Could you check a few things on this model? Use its own coordinates, in mm. A direction names the side the tool comes from. Round coordinates to 2 decimals unless told otherwise and drop trailing zeros. Loops run counter-clockwise (first coordinate to the right, second up) from the corner with the lowest first, then second, coordinate; pieces in that order, holes last. Notation, with made-up numbers: (-18, 56.5) - (1, 56.5) arc R21 ccw to (1, 81.5) - close; hole circle Ø7 at (84.5, 9.5). An arc over 180 degrees is marked (long way). Put each result on its own line as item: value. Start each with the question number.
from build123d import *

# Parameters (mm, degrees)
SKETCH1_R               = 75
BOSS_EXTRUDE1_DEPTH     = 50
CUT_EXTRUDE1_DEPTH      = 290.39592257
CUT_EXTRUDE1_DEPTH_BACK = 290.39592257
FILLET1_START           = -50
FILLET1_DEPTH           = 100


with BuildPart() as part:
    # Sketch1 → Boss-Extrude1 (new, symmetric)
    with BuildSketch(Plane.XY):
        with BuildLine():
            Line((-95.945006832, -117.34375), (-36.550478793, 16.25))
            ThreePointArc((-36.550478793, 16.25), (0, 40), (36.550478793, 16.25))
            Line((36.550478793, 16.25), (95.945006832, -117.34375))
            ThreePointArc((95.945006832, -117.34375), (0, -265), (-95.945006832, -117.34375))
        make_face()
        with Locations((0, -160)):
            Circle(SKETCH1_R, mode=Mode.SUBTRACT)
    extrude(amount=BOSS_EXTRUDE1_DEPTH, both=True)

    # Sketch2 → Cut-Extrude1 (cut, two sides: drawn at the far end of the back side and taken through both)
    with BuildSketch(Plane.XY.offset(-CUT_EXTRUDE1_DEPTH_BACK)):
        with BuildLine():
            Line((-35.52920143, -18.375958363), (-82.238577284, -123.4375))
            ThreePointArc((-82.238577284, -123.4375), (0, -70), (82.238577284, -123.4375))
            Line((82.238577284, -123.4375), (35.52920143, -18.375958363))
            ThreePointArc((35.52920143, -18.375958363), (0, -40), (-35.52920143, -18.375958363))
        make_face()
    extrude(amount=CUT_EXTRUDE1_DEPTH + CUT_EXTRUDE1_DEPTH_BACK, mode=Mode.SUBTRACT)

    # Fillet1: read off the stored shape, not the designer's step
    # Fillet1 outline → Fillet1 (add)
    with BuildSketch(Plane.XY.offset(FILLET1_START)):
        with BuildLine():
            ThreePointArc((-42.220939274, -33.427418189), (-35.213916082, -27.719526256), (-26.466655661, -29.991934551))
            ThreePointArc((-26.466655661, -29.991934551), (-31.537347698, -24.604790188), (-35.52920143, -18.375958363))
            Line((-35.52920143, -18.375958363), (-42.220939274, -33.427418189))
        make_face()
        with BuildLine():
            ThreePointArc((35.52920143, -18.375958363), (31.537347698, -24.604790188), (26.466655661, -29.991934551))
            ThreePointArc((26.466655661, -29.991934551), (35.213916082, -27.719526256), (42.220939274, -33.427418189))
            Line((42.220939274, -33.427418189), (35.52920143, -18.375958363))
        make_face()
        with BuildLine():
            ThreePointArc((-43.853361827, -81.406853629), (-55.469552548, -80.058313703), (-57.863577284, -68.61178181))
            Line((-57.863577284, -68.61178181), (-82.238577284, -123.4375))
            ThreePointArc((-82.238577284, -123.4375), (-66.45628703, -99.30764534), (-43.853361827, -81.406853629))
        make_face()
        with BuildLine():
            Line((82.238577284, -123.4375), (57.863577284, -68.61178181))
            ThreePointArc((57.863577284, -68.61178181), (55.469552548, -80.058313703), (43.853361827, -81.406853629))
            ThreePointArc((43.853361827, -81.406853629), (66.45628703, -99.30764534), (82.238577284, -123.4375))
        make_face()
    extrude(amount=FILLET1_DEPTH)


solid = part.part
Item 1: Thinking about a two-plate mould opening in X: for faces 1 (the face through (55.598, -79.939, -0.7)), 2 (the face through (65.83, -49.61, 0.7)), 3 (the face through (0, -78, 50)), which applies, released by +X, released by -X, zero draft, split by the parting line, or undercut?
Item 2: Suppose I cut it at B-B, the plane x = 0. List the corners of the cut face in (y, z) for me, then the cut area to 3 significant figures.
Item 3: Will these pins go through, and if not, where does the flat tip stop? P1, Ø1.5, axis at y = -122.5, z = 34.5, coming from the -X side; P2, Ø8, axis at y = -197.5, z = -9.5, coming from the -X side.
Item 4: I need wall thicknesses on line 1 (Y direction, x = -11, z = -37.5); line 2 (Y direction, x = -51.5, z = 14); line 3 (X direction, y = -125, z = 14.5). Which ranges of each line are inside material? Lowest first, please. Write a range as from..to.
Item 5: Suppose I cut it at D-D, the plane y = -110. List the corners of the cut face in (x, z) for me.
Item 6: Suppose I cut it at A-A, the plane z = 3.5. List the corners of the cut face in (x, y) for me (3 decimals), then the cut area to 3 significant figures.
Item 7: Suppose I cut it at C-C, the plane y = -160. List the corners of the cut face in (x, z) for me, then the cut area to 3 significant figures.
Item 8: On a 3-axis mill with a long thin cutter (end or side, diameter ignored), from which of +Z, -Z, +X, -X, +Y, -Y can I reach the whole of each face in a straight line? I mean faces 4 (the face through (35.085, -27.692, -0.7)), 5 (the face through (0, -78, -50)). Say none if no direction works.
Numbers:
1. face 1: undercut
1. face 2: released by +X
1. face 3: zero draft
2. outline: (-265, -50) - (-235, -50) - (-235, 50) - (-265, 50) - close; (-85, -50) - (-70, -50) - (-70, 50) - (-85, 50) - close; (-40, -50) - (40, -50) - (40, 50) - (-40, 50) - close
2. area: 12,500 mm^2
3. P1: x = -98.36
3. P2: x = -99.51
4. line 1: -264.42..-234.19, -85.81..-70.67, -38.46..38.46
4. line 2: -251.5..-214.52, -105.48..-82.28, -54.3..-17.38
4. line 3: -98.99..-66.33, 66.33..98.99
5. outline: (-92.68, -50) - (-55.9, -50) - (-55.9, 50) - (-92.68, 50) - close; (55.9, -50) - (92.68, -50) - (92.68, 50) - (55.9, 50) - close
6. outline: (-95.945, -117.344) arc R105 ccw (long way) to (95.945, -117.344) - (36.55, 16.25) arc R40 ccw to (-36.55, 16.25) - close; hole circle Ø150 at (0, -160); hole (-57.864, -68.612) arc R10 ccw to (-43.853, -81.407) arc R90 cw to (43.853, -81.407) arc R10 ccw to (57.864, -68.612) - (42.221, -33.427) arc R10 ccw to (26.467, -29.992) arc R40 cw to (-26.467, -29.992) arc R10 ccw to (-42.221, -33.427) - close
6. area: 23,000 mm^2
7. outline: (-105, -50) - (-75, -50) - (-75, 50) - (-105, 50) - close; (75, -50) - (105, -50) - (105, 50) - (75, 50) - close
7. area: 6,000 mm^2
8. face 4: +Z, -Z
8. face 5: -Z, +X, -X, +Y, -Y
